Geometry: final body of the model. Coordinates: model frame, mm. A direction names the side the tool comes from. Round coordinates to 2 decimals unless told otherwise and drop trailing zeros. Write each loop counter-clockwise with the first axis right and the second up, starting at its lowest first coordinate (ties: lowest second). Pieces come first, ordered by that corner, then holes. Notation, with made-up numbers: M 63,53 L 68,53 A26 cw 68,82 Z; hole C 0,-36.5 d3. An arc over 180 degrees is marked long. Put each result on its own line as item: value. Start each with the question number.
```python
from build123d import *

# Parameters (mm, degrees)
SKETCH1_R           = 32.5
BOSS_EXTRUDE1_DEPTH = 26
FILLET1_R           = 2.54
SKETCH2_R           = 3.1115
CUT_EXTRUDE1_DEPTH  = 26
SKETCH3_R           = 14.2875
CUT_EXTRUDE2_DEPTH  = 13.97


with BuildPart() as part:
    # Sketch1 → Boss-Extrude1 (new body)
    with BuildSketch(Plane.XY):
        with Locations(Location((0, 0, 0), (0, 0, 180))):
            Circle(SKETCH1_R)
    extrude(amount=BOSS_EXTRUDE1_DEPTH)

    # Fillet1
    fillet1_edges = [part.edges().sort_by_distance(p)[0] for p in [
        (32.5, 0, 0),
        (32.5, 0, 26),
    ]]
    fillet(fillet1_edges, radius=FILLET1_R)

    # Sketch2 → Cut-Extrude1 (cut)
    with BuildSketch(Plane.XY.offset(26)):
        Circle(SKETCH2_R)
    extrude(amount=-CUT_EXTRUDE1_DEPTH, mode=Mode.SUBTRACT)

    # Sketch3 → Cut-Extrude2 (cut)
    with BuildSketch(Plane.XY.offset(26)):
        Circle(SKETCH3_R)
    extrude(amount=-CUT_EXTRUDE2_DEPTH, mode=Mode.SUBTRACT)


solid = part.part
```
1) Draft query along Y for faces 1 (the face through (-14.274, 0.628, 19.113)), 2 (the face through (0, 6, 0)), 3 (the face through (-31, -9.76, 12.85)), 4 (the face through (-0.67, -3.04, 6.1)). Return one class per face: +Y half, -Y half, draft (parallel to the pull), parting line (faces both ways), or undercut.
2) Section A-A, the plane x = 0. Output: boundary loops of the cut face in (y, z), and give its area (3 significant figures).
3) Access query for faces 5 (the face through (-0.2, 3.4, 12.03)), 6 (the face through (-13, -7, 26)). Directions: +Z, -Z, +X, -X, +Y, -Y. A direction counts if a zero-diameter tool reaches every point of the face in a straight line with its end or side. Return the directions, or none.
4) Ray query, probe 1 along Y at (x, z) = (0, 16.75); probe 2 along Z at (x, y) = (8.5, -5); probe 3 along Y at (x, z) = (2, 24.5). Return the intervals inside material, ascending.
5) First-contact query: pin 1 (14.5 mm diameter, centred on x = 5, y = 1, fed in from +Z); pin 2 (2 mm diameter, centred on y = 13.5, z = 17.5, fed in from -X); pin 3 (2 mm diameter, centred on x = 6.5, y = 14, fed in from -Z); pin 4 (1.5 mm diameter, centred on x = -22, z = 10.5, fed in from +Y). Flat tips, straight axial feed; report the tip coordinate or a pass-through.
6) Section C-C, the plane z = 13.5. Output: boundary loops of the cut face in (x, y) (1 decimal).
7) Section D-D, the plane z = 9.75. Output: boundary loops of the cut face in (x, y), and give its area (3 significant figures).
Solved:
1. face 1: undercut
1. face 2: draft
1. face 3: parting line
1. face 4: undercut
2. outline: M -32.5,2.54 A2.54 ccw -29.96,0 L -3.11,0 L -3.11,12.03 L -14.29,12.03 L -14.29,26 L -29.96,26 A2.54 ccw -32.5,23.46 Z; M 3.11,0 L 29.96,0 A2.54 ccw 32.5,2.54 L 32.5,23.46 A2.54 ccw 29.96,26 L 14.29,26 L 14.29,12.03 L 3.11,12.03 Z
2. area: 1,210 mm2
3. face 5: +Z
3. face 6: +Z, +X, -X, +Y, -Y
4. probe 1: y = -32.5 to -14.29, 14.29 to 32.5
4. probe 2: z = 0 to 12.03
4. probe 3: y = -32.22 to -14.15, 14.15 to 32.22
5. pin 1: stops at z = 12.03
5. pin 2: stops at x = -30
5. pin 3: stops at z = 0
5. pin 4: stops at y = 24.59
6. outline: C 0,0 d65; hole C 0,0 d28.6
7. outline: C 0,0 d65; hole C 0,0 d6.22
7. area: 3,290 mm2
